For this review, take the finished solid that the model builds, in its own axes (mm). A direction names the side the tool comes from. Give positions to 0.01 mm unless a question says otherwise; leave off trailing zeros. Loops run counter-clockwise (first coordinate to the right, second up) from the corner with the lowest first, then second, coordinate; pieces in that order, holes last. Notation, with made-up numbers: (-23.75, 69) -> (30.25, 69) arc R28 ccw to (30.25, 108) -> close; hole circle Ø6 at (11, 74.25). An arc over 180 degrees is marked (long way). Write each question's results on one line, items separated by ' | '. Start each with the question number.
```python
from build123d import *

# Parameters (mm, degrees)
ESBO_O1_R                = 5.145
RESSALTO_EXTRUS_O1_DEPTH = 3
ESBO_O2_R                = 1.75
CORTE_EXTRUS_O1_DEPTH    = 4
FILETE1_R                = 1.5
ESBO_O3_R                = 3.7
RESSALTO_EXTRUS_O2_DEPTH = 4.2
ESBO_O4_R                = 2.2
CORTE_EXTRUS_O2_DEPTH    = 4.2


with BuildPart() as part:
    # Esboço1 → Ressalto-extrusão1 (new body)
    with BuildSketch(Plane(origin=(0, 0, 0), x_dir=(1, 0, 0), z_dir=(0, 1, 0))):
        Polygon((-55.63, 45.795), (-55.63, 84.055), (55.63, 84.055), (55.63, -84.055), (-55.63, -84.055), (-55.63, 32.315), (-51.63, 32.315), (-51.63, 45.795), align=None)
        with Locations((2.13, -42.945)):
            Circle(ESBO_O1_R, mode=Mode.SUBTRACT)
        with BuildLine():
            Line((0.63, -53.125083497), (0.63, -50.511755976))
            ThreePointArc((0.63, -50.511755976), (-3.32462171, -48.39962171), (-5.436755976, -44.445))
            Line((-5.436755976, -44.445), (-8.050083497, -44.445))
            ThreePointArc((-8.050083497, -44.445), (-5.146128778, -50.221128778), (0.63, -53.125083497))
        make_face(mode=Mode.SUBTRACT)
        with BuildLine():
            Line((0.63, -60.882391115), (0.63, -55.717219854))
            ThreePointArc((0.63, -55.717219854), (-6.963393206, -52.038393206), (-10.642219854, -44.445))
            Line((-10.642219854, -44.445), (-15.807391115, -44.445))
            ThreePointArc((-15.807391115, -44.445), (-10.597922061, -55.672922061), (0.63, -60.882391115))
        make_face(mode=Mode.SUBTRACT)
        with BuildLine():
            Line((3.63, -60.882391115), (3.63, -55.717219854))
            ThreePointArc((3.63, -55.717219854), (11.223393206, -52.038393206), (14.902219854, -44.445))
            Line((14.902219854, -44.445), (20.067391115, -44.445))
            ThreePointArc((20.067391115, -44.445), (14.857922061, -55.672922061), (3.63, -60.882391115))
        make_face(mode=Mode.SUBTRACT)
        with BuildLine():
            Line((3.63, -53.125083497), (3.63, -50.511755976))
            ThreePointArc((3.63, -50.511755976), (7.58462171, -48.39962171), (9.696755976, -44.445))
            Line((9.696755976, -44.445), (12.310083497, -44.445))
            ThreePointArc((12.310083497, -44.445), (9.406128778, -50.221128778), (3.63, -53.125083497))
        make_face(mode=Mode.SUBTRACT)
        with BuildLine():
            Line((14.902219854, -41.445), (20.067391115, -41.445))
            ThreePointArc((20.067391115, -41.445), (14.857922061, -30.217077939), (3.63, -25.007608885))
            Line((3.63, -25.007608885), (3.63, -30.172780146))
            ThreePointArc((3.63, -30.172780146), (11.223393206, -33.851606794), (14.902219854, -41.445))
        make_face(mode=Mode.SUBTRACT)
        with BuildLine():
            Line((-15.807391115, -41.445), (-10.642219854, -41.445))
            ThreePointArc((-10.642219854, -41.445), (-6.963393206, -33.851606794), (0.63, -30.172780146))
            Line((0.63, -30.172780146), (0.63, -25.007608885))
            ThreePointArc((0.63, -25.007608885), (-10.597922061, -30.217077939), (-15.807391115, -41.445))
        make_face(mode=Mode.SUBTRACT)
        with BuildLine():
            Line((-8.050083497, -41.445), (-5.436755976, -41.445))
            ThreePointArc((-5.436755976, -41.445), (-3.32462171, -37.49037829), (0.63, -35.378244024))
            Line((0.63, -35.378244024), (0.63, -32.764916503))
            ThreePointArc((0.63, -32.764916503), (-5.146128778, -35.668871222), (-8.050083497, -41.445))
        make_face(mode=Mode.SUBTRACT)
        with BuildLine():
            Line((3.63, -35.378244024), (3.63, -32.764916503))
            ThreePointArc((3.63, -32.764916503), (9.406128778, -35.668871222), (12.310083497, -41.445))
            Line((12.310083497, -41.445), (9.696755976, -41.445))
            ThreePointArc((9.696755976, -41.445), (7.58462171, -37.49037829), (3.63, -35.378244024))
        make_face(mode=Mode.SUBTRACT)
    extrude(amount=RESSALTO_EXTRUS_O1_DEPTH)

    # Esboço2 → Corte-extrusão1 (cut, through all)
    with BuildSketch(Plane(origin=(0, 3, 0), x_dir=(1, 0, 0), z_dir=(0, 1, 0))):
        with Locations((-52.37, -74.445)):
            Circle(ESBO_O2_R)
        with Locations((50.63, -74.445)):
            Circle(ESBO_O2_R)
        with BuildLine():
            Line((-1.47, 55.855), (2.73, 55.855))
            ThreePointArc((2.73, 55.855), (4.53, 54.055), (2.73, 52.255))
            Line((2.73, 52.255), (-1.47, 52.255))
            ThreePointArc((-1.47, 52.255), (-3.27, 54.055), (-1.47, 55.855))
        make_face()
    extrude(amount=-CORTE_EXTRUS_O1_DEPTH, mode=Mode.SUBTRACT)

    # Filete1
    filete1_edges = [part.edges().sort_by_distance(p)[0] for p in [
        (-51.63, 1.5, -45.795),
        (-55.63, 1.5, -45.795),
        (-55.63, 1.5, -84.055),
        (55.63, 1.5, -84.055),
        (55.63, 1.5, 84.055),
        (-55.63, 1.5, 84.055),
        (-55.63, 1.5, -32.315),
        (-51.63, 1.5, -32.315),
    ]]
    fillet(filete1_edges, radius=FILETE1_R)

    # Esboço3 → Ressalto-extrusão2 (add)
    with BuildSketch(Plane.XZ):
        with Locations((18.13, 26.945)):
            Circle(ESBO_O3_R)
        with Locations((18.13, 58.945)):
            Circle(ESBO_O3_R)
        with Locations((-13.87, 58.945)):
            Circle(ESBO_O3_R)
        with Locations((-13.87, 26.945)):
            Circle(ESBO_O3_R)
    extrude(amount=RESSALTO_EXTRUS_O2_DEPTH)

    # Esboço4 → Corte-extrusão2 (cut)
    with BuildSketch(Plane.XZ.offset(4.2)):
        with Locations((-13.87, 58.945)):
            Circle(ESBO_O4_R)
        with Locations((18.13, 58.945)):
            Circle(ESBO_O4_R)
        with Locations((18.13, 26.945)):
            Circle(ESBO_O4_R)
        with Locations((-13.87, 26.945)):
            Circle(ESBO_O4_R)
    extrude(amount=-CORTE_EXTRUS_O2_DEPTH, mode=Mode.SUBTRACT)


solid = part.part
```
1. Wall thickness on L1, parallel to Z at x = 18.13, y = -2.3 (3 decimals); L2, parallel to Z at x = -52.37, y = 1.65 (3 decimals); L3, parallel to X at y = 1, z = 57.5: over which ranges is each line inside the solid? List them lowest first.
2. We need section B-B (x = 50.63). Write out the cut boundary in (y, z) (3 decimals), plus the area to 3 significant figures.
3. We need section C-C (x = -13.87). Write out the cut boundary in (y, z) (3 decimals).
4. We need section A-A (y = -1.25). Write out the cut boundary in (x, z) (3 decimals), plus the area to 3 significant figures.
5. Draft analysis for pull direction X (two halves, no side actions). For faces 3 (the cylindrical face through (11.14, 1.48, 33.77)), 4 (the flat face through (20, -4.2, 57)), state which applies: released by +X, released by -X, zero draft, split by the parting line, or undercut.
6. We need section D-D (z = -29). Write out the cut boundary in (x, y), plus the area to 3 significant figures.
7. For pin 1 Ø2 at (x, z) = (-17, -49) entering from -Y, flat-tipped, find the tip position at first contact; note if it passes through.
8. Machinability: for faces 1 (the flat face through (-14, 0, 59)), 2 (the cylindrical face through (50.4, 1.52, 72.71)), which of the approach directions +Z, -Z, +X, -X, +Y, -Y give a long, thin tool a straight path to every point of the face, cutting with its end or side? Answer none if there is none.
Response:
1) L1: z = 23.245 to 24.745, 29.145 to 30.645, 55.245 to 56.745, 61.145 to 62.645 | L2: z = -84.055 to -45.588, -32.522 to 72.695, 76.195 to 84.055 | L3: x = -55.63 to -8.46, 0.63 to 3.63, 12.72 to 55.63
2) outline: (0, -84.055) -> (3, -84.055) -> (3, 72.695) -> (0, 72.695) -> close; (0, 76.195) -> (3, 76.195) -> (3, 84.055) -> (0, 84.055) -> close | area: 494 mm2
3) outline: (-4.2, 23.245) -> (0, 23.245) -> (0, -84.055) -> (3, -84.055) -> (3, 34.699) -> (0, 34.699) -> (0, 30.645) -> (-4.2, 30.645) -> (-4.2, 29.145) -> (0, 29.145) -> (0, 24.745) -> (-4.2, 24.745) -> close; (-4.2, 55.245) -> (0, 55.245) -> (0, 51.191) -> (3, 51.191) -> (3, 84.055) -> (0, 84.055) -> (0, 62.645) -> (-4.2, 62.645) -> (-4.2, 61.145) -> (0, 61.145) -> (0, 56.745) -> (-4.2, 56.745) -> close; (0, 41.445) -> (3, 41.445) -> (3, 44.445) -> (0, 44.445) -> close
4) outline: circle Ø7.4 at (-13.87, 26.945); circle Ø7.4 at (-13.87, 58.945); circle Ø7.4 at (18.13, 26.945); circle Ø7.4 at (18.13, 58.945); hole circle Ø4.4 at (-13.87, 26.945); hole circle Ø4.4 at (-13.87, 58.945); hole circle Ø4.4 at (18.13, 26.945); hole circle Ø4.4 at (18.13, 58.945) | area: 111 mm2
5) face 3: undercut | face 4: zero draft
6) outline: (-55.63, 0) -> (55.63, 0) -> (55.63, 3) -> (-55.63, 3) -> close | area: 334 mm2
7) pin 1: stops at y = 0
8) face 1: -Y | face 2: +Y, -Y
